Check sheet for the modelled part. Datum: model origin and axes. Units: mm. Round coordinates to 2 decimals unless told otherwise and drop trailing zeros. Write each loop counter-clockwise with the first axis right and the second up, starting at its lowest first coordinate (ties: lowest second). Pieces come first, ordered by that corner, then holes. Notation, with made-up numbers: (-21.5, 89) -> (-10.5, 89) arc R6 cw to (-10.5, 98) -> close; hole circle Ø11 at (63, 26.25). An arc over 180 degrees is marked (long way). One line per item, written item: value.
Autodesk Inventor part; units mm, degrees
ref_plane "YZ Plane" through (0, 0, 0) normal (1, 0, 0) x (0, 1, 0)
ref_plane "XZ Plane" through (0, 0, 0) normal (0, 1, 0) x (-1, 0, 0)
ref_plane "XY Plane" through (0, 0, 0) normal (0, 0, 1) x (1, 0, 0)
sketch "Sketch1" plane through (0, 0, 0) normal (0, 1, 0) x (-1, 0, 0)
  line L0 (45, -45) -> (-45, -45)
  line L1 (-45, -45) -> (-45, 45)
  line L2 (-45, 45) -> (45, 45)
  line L3 (45, 45) -> (45, -45)
  line L4 (45, -45) -> (-45, 45) construction
  line L5 (-45, -45) -> (45, 45) construction
  point P0 (0, 0)
  dimension "d2" = 90
  dimension "d3" = 90
extrude "Extrusion1" add sketch "Sketch1" along normal blind 2
sketch "Sketch2" plane through (0, 2, 0) normal (0, 1, 0) x (1, 0, 0)
  line L0 (45, -45) -> (45, 45)
  line L1 (45, 45) -> (41, 45)
  line L2 (45, 45) -> (-45, 45)
  circle A0 centre (41, 41) radius 2
  point P0 (0, 0)
hole "Hole1" at (41, 2, -41) direction (0, -1, 0) diameter 4 end through all
sketch "Sketch3" plane through (0, 2, 0) normal (0, 1, 0) x (1, 0, 0)
  circle A0 centre (-41, 41) radius 2
  line L0 (-45, 45) -> (-45, -45)
  circle A1 centre (-41, -41) radius 2
  line L1 (45, -45) -> (45, 45)
  circle A2 centre (41, -41) radius 2
  point P0 (0, 0)
  dimension "d17" = 4
  dimension "d21" = 4
extrude "Extrusion2" cut sketch "Sketch3" against normal blind 2
fillet "Fillet1" radius 3.5 4 edges at (-45, 1, -45) (45, 1, -45) (45, 1, 45) (-45, 1, 45)
sketch "Sketch5" plane through (0, 2, 0) normal (0, 1, 0) x (1, 0, 0)
  line L0 (40, 40) -> (-40, 40)
  line L1 (-40, 40) -> (-40, -40)
  line L2 (-40, -40) -> (40, -40)
  line L3 (40, -40) -> (40, 40)
  line L4 (40, 40) -> (-40, -40) construction
  line L5 (-40, 40) -> (40, -40) construction
  line L6 (-9.8412, 41.25) -> (-37.3412, 41.25)
  line L7 (-37.3412, 41.25) -> (-37.3412, -41.25)
  line L8 (-37.3412, -41.25) -> (-9.8412, -41.25)
  line L9 (-9.8412, -41.25) -> (-9.8412, 41.25)
  line L10 (-9.8412, 41.25) -> (-37.3412, -41.25) construction
  line L11 (-37.3412, 41.25) -> (-9.8412, -41.25) construction
  line L12 (26.1588, 41.25) -> (-6.3412, 41.25)
  line L13 (-6.3412, 41.25) -> (-6.3412, -41.25)
  line L14 (-6.3412, -41.25) -> (26.1588, -41.25)
  line L15 (26.1588, -41.25) -> (26.1588, 41.25)
  line L16 (26.1588, 41.25) -> (-6.3412, -41.25) construction
  line L17 (-6.3412, 41.25) -> (26.1588, -41.25) construction
  line L18 (37.1268, 41.25) -> (29.6588, 41.25)
  line L19 (29.6588, 41.25) -> (29.6588, -41.25)
  line L20 (29.6588, -41.25) -> (37.1268, -41.25)
  line L21 (37.1268, -41.25) -> (37.1268, 41.25)
  line L22 (37.1268, 41.25) -> (29.6588, -41.25) construction
  line L23 (29.6588, 41.25) -> (37.1268, -41.25) construction
  line L24 (-41.5049, 41.25) -> (-37.5049, 41.25)
  line L25 (41.2164, 37.1336) -> (36.7164, 37.1336)
  line L26 (36.7164, 37.1336) -> (36.7164, -36.7164)
  line L27 (36.7164, -36.7164) -> (41.2164, -36.7164)
  line L28 (41.2164, -36.7164) -> (41.2164, 37.1336)
  line L29 (41.2164, 37.1336) -> (36.7164, -36.7164) construction
  line L30 (36.7164, 37.1336) -> (41.2164, -36.7164) construction
  line L31 (37.1268, 41.25) -> (41.1268, 41.25)
  line L32 (41.1268, 41.25) -> (41.1268, 37.25)
  point P0 (0, 0)
  point P1 (-23.5912, 0)
  point P2 (9.9088, 0)
  point P3 (33.3928, 0)
  point P4 (38.9664, 0.2086)
  point P5 (37.1268, 37.1336)
  point P6 (37.1268, 40)
  point P7 (29.6588, 40)
  point P8 (29.6588, -40)
  point P9 (37.1268, -40)
  point P10 (37.1268, -36.7164)
  dimension "d25" = 80
  dimension "d26" = 80
  dimension "d27" = 27.5
  dimension "d28" = 82.5
  dimension "d29" = 32.5
  dimension "d30" = 82.5
  dimension "d31" = 7.468
  dimension "d32" = 82.5
  dimension "d33" = 4
  dimension "d34" = 3.5
  dimension "d35" = 3.5
  dimension "d36" = 4.5
  dimension "d37" = 4
  dimension "d38" = 4
  dimension "d39" = 73.85
extrude "Extrusion4" cut sketch "Sketch5" against normal through all contours L21 L25 L26 L27 L2 L19 L0 | L0 L19 L18 L21 | L25 L28 L27 L3 | L3 L27 L21 L25 | L21 L27 L26 L25 | L15 L2 L13 L0 | L0 L13 L12 L15 | L2 L21 L20 L19 | L15 L14 L13 L2 | L9 L2 L7 L0 | L0 L7 L6 L9 | L9 L8 L7 L2
sketch "Sketch8" plane through (0, 2, 0) normal (0, 1, 0) x (1, 0, 0)
  line L0 (-45, 41.5) -> (-45, -41.5)
  line L1 (-45, 41.5) -> (-44, 41.5)
  line L2 (41.5, 45) -> (-41.5, 45)
  line L3 (-41.5, 45) -> (-41.5, 44)
  line L4 (-45, -41.5) -> (-44, -41.5)
  arc A0 (-45, -41.5) -> (-41.5, -45) centre (-41.5, -41.5) ccw
  line L5 (-41.5, -45) -> (-41.5, -44)
  line L6 (41.5, -45) -> (41.5, -44)
  arc A1 (41.5, -45) -> (45, -41.5) centre (41.5, -41.5) ccw
  line L7 (45, -41.5) -> (44, -41.5)
  arc A2 (45, 41.5) -> (41.5, 45) centre (41.5, 41.5) ccw
  circle A3 centre (-41, -41) radius 2
  line L8 (-41, -39) -> (-41, -38)
  line L9 (-39, -41) -> (-38, -41)
  circle A4 centre (-41, 41) radius 2
  line L10 (-39, 41) -> (-38, 41)
  line L11 (-41, 39) -> (-41, 38)
  circle A5 centre (41, 41) radius 2
  line L12 (37.1268, 41.25) -> (37.1268, 37.1336)
  circle A6 centre (41, -41) radius 2
  line L13 (41, -39) -> (41, -38)
  line L14 (39, -41) -> (38, -41)
  line L15 (-44, 37.3438) -> (-41.5, 37.3438)
  line L16 (-41.5, 37.3438) -> (-41.5, -37.5309)
  line L17 (-41.5, -37.5309) -> (-44, -37.5309)
  line L18 (-44, -37.5309) -> (-44, 37.3438)
  line L19 (37.5845, -44) -> (-37.7671, -44)
  line L20 (-37.7671, -44) -> (-37.7671, -41.5)
  line L21 (-37.7671, -41.5) -> (37.5845, -41.5)
  line L22 (37.5845, -41.5) -> (37.5845, -44)
  line L23 (44, 34.9904) -> (41.5, 34.9904)
  line L24 (41.5, 34.9904) -> (41.5, -37.4955)
  line L25 (41.5, -37.4955) -> (44, -37.4955)
  line L26 (44, -37.4955) -> (44, 34.9904)
  line L27 (-37.4232, 44) -> (37.7379, 44)
  line L28 (37.7379, 44) -> (37.7379, 41.5)
  line L29 (37.7379, 41.5) -> (-37.4232, 41.5)
  line L30 (-37.4232, 41.5) -> (-37.4232, 44)
  line L31 (26.1588, -41.5) -> (28.1588, -41.5)
  line L32 (28.1588, -41.5) -> (28.1588, 41.5)
  line L33 (28.1588, 41.5) -> (26.1588, 41.5)
  line L34 (26.1588, 41.5) -> (26.1588, -41.5)
  line L35 (-9.8412, -41.5) -> (-7.8412, -41.5)
  line L36 (-7.8412, -41.5) -> (-7.8412, 41.5)
  line L37 (-7.8412, 41.5) -> (-9.8412, 41.5)
  line L38 (-9.8412, 41.5) -> (-9.8412, -41.5)
  point P0 (0, 0)
  dimension "d46" = 1
  dimension "d47" = 1
  dimension "d48" = 1
  dimension "d49" = 1
  dimension "d50" = 1
  dimension "d51" = 1
  dimension "d54" = 1
  dimension "d55" = 1
  dimension "d56" = 1
  dimension "d57" = 1
  dimension "d60" = 1
  dimension "d61" = 1
  dimension "d63" = 2.5
  dimension "d64" = 2.5
  dimension "d65" = 2.5
  dimension "d72" = 2
  dimension "d73" = 2
extrude "Extrusion5" add sketch "Sketch8" along normal blind 5 contours L15 L16 L17 L18 | L19 L20 L21 L22 | L21 L34 L29 L32 | L38 L29 L36 L21 | L29 L30 L27 L28 | L26 L25 L24 L23
fillet "Fillet3" radius 3.5 1 edges at (37.1268, 1, 36.7164)
fillet "Fillet4" radius 3.5 8 edges at (-6.3412, 1, 41.25) (-6.3412, 1, -41.25) (29.6588, 1, -41.25) (29.6588, 1, 41.25) (26.1588, 1, -41.25) (-9.8412, 1, -41.25) (26.1588, 1, 41.25) (-9.8412, 1, 41.25)
fillet "Fillet7" radius 1 4 edges at (-7.8412, 4.5, 41.5) (28.1588, 4.5, 41.5) (26.1588, 4.5, 41.5) (-9.8412, 4.5, 41.5)
sketch "Sketch10" plane through (0, 0, 0) normal (0, -1, 0) x (1, 0, 0)
  line L0 (-37.3412, -41.25) -> (-37.3412, 41.25)
  line L1 (-37.3412, 37.75) -> (-40.8412, 37.75)
  line L2 (-40.8412, 37.75) -> (-40.8412, -37)
  line L3 (-40.8412, -37) -> (-37.3412, -37)
  line L4 (-37.3412, -37) -> (-37.3412, 37.75)
  point P0 (0, 0)
  point P1 (-37.3412, -37.75)
  dimension "d78" = 3.5
extrude "Extrusion6" cut sketch "Sketch10" against normal through all
fillet "Fillet8" radius 3.5 1 edges at (-37.3412, 1, -37)
fillet "Fillet11" radius 3.5 2 edges at (37.1268, 1, -37.1336) (-37.3412, 1, 37.75)
sketch "Sketch19" plane through (-37.7671, 2, 44) normal (0, 0, 1) x (1, 0, 0)
  line L0 (75.3516, 0) -> (0, 0)
  line L1 (0, 5) -> (75.3516, 5)
  line L2 (0, 0) -> (0, 5)
  line L3 (0, 5) -> (0, 3)
  line L4 (0, 3) -> (1.2108, 3)
  line L5 (1.2108, 3) -> (1.2108, 5)
  line L6 (1.2108, 5) -> (0, 5)
  line L7 (0, 5) -> (0, 3)
  point P0 (37.7671, -2)
  dimension "d90" = 2
  dimension "d106" = 1.2108
extrude "Extrusion7" cut sketch "Sketch19" against normal blind 3
sketch "Sketch21" plane through (25.1588, 2, 41.5) normal (0, 0, -1) x (-1, 0, 0)
  line L0 (32, 0) -> (0, 0)
  line L1 (0, 5) -> (32, 5)
  line L2 (28.159, 5) -> (29.959, 5)
  line L3 (29.959, 5) -> (29.959, 4)
  line L4 (28.159, 5) -> (26.359, 5)
  line L5 (29.959, 5) -> (26.359, 5)
  line L6 (26.359, 5) -> (26.359, 3)
  line L7 (26.359, 3) -> (29.959, 3)
  line L8 (29.959, 3) -> (29.959, 5)
  point P0 (25.1588, -2)
  point P1 (29.959, 4)
  dimension "d102" = 1.8
  dimension "d103" = 1
  dimension "d104" = 1.8
  dimension "d105" = 2
extrude "Extrusion8" cut sketch "Sketch21" against normal up to surface (2.5 mm away)
sketch "Sketch22" plane through (-9.8412, 2, -41.5) normal (-1, 0, 0) x (0, 0, 1)
  line L0 (0, 5) -> (82, 5)
  line L1 (0, 5) -> (3, 5)
  line L2 (3.75, 0) -> (0, 0)
  line L3 (3, 5) -> (0, 5)
  line L4 (0, 5) -> (0, 0)
  line L5 (0, 0) -> (3, 0)
  line L6 (3, 0) -> (3, 5)
  point P0 (41.5, -2)
  point P1 (3, 0)
  dimension "d98" = 3
extrude "Extrusion9" cut sketch "Sketch22" against normal up to surface (38 mm away)
sketch "Sketch23" plane through (-37.7671, 2, 44) normal (0, 0, 1) x (1, 0, 0)
  line L0 (33.7518, 5) -> (31.9518, 5)
  line L1 (36.5669, 5) -> (75.3516, 5)
  line L2 (31.9518, 5) -> (31.9518, 3.1171)
  point P0 (37.7671, -2)
  point P1 (0.3379, 5)
  dimension "d101" = 1.8
sketch "Sketch24" plane through (-37.7671, 2, 44) normal (0, 0, 1) x (1, 0, 0)
  point P0 (37.7671, -2)
properties part number "LeftCover" material "ABS Plastic"
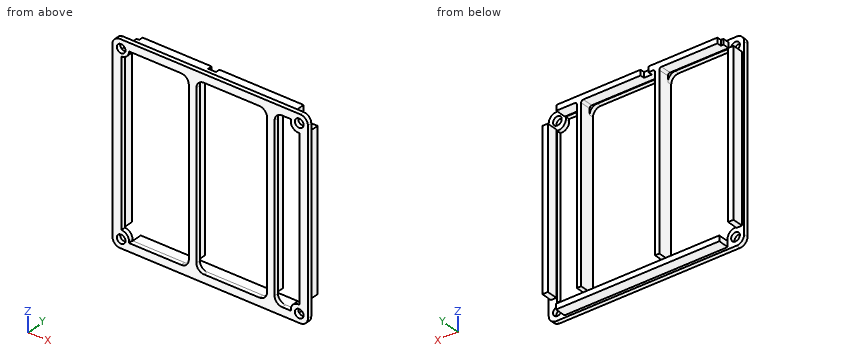
Item 1: Sectioned sample at B-B on x = 18. Enter the section's corners in (y, z), and give its area (3 significant figures).
Answer:
outline: (0, -45) -> (2, -45) -> (2, -44) -> (7, -44) -> (7, -41.5) -> (2, -41.5) -> (2, -41.25) -> (0, -41.25) -> close; (0, 41.25) -> (2, 41.25) -> (2, 41.5) -> (7, 41.5) -> (7, 44) -> (2, 44) -> (2, 45) -> (0, 45) -> close
area: 40.0 mm^2
Item 2: Depth check by flat-ended pin: P1, Ø6, axis at x = -35.5, z = -0.5, coming from the +Y side (3 decimals); P2, Ø1.2, axis at y = 3.5, z = -42.5, coming from the -X side; P3, Ø2, axis at x = -42.5, y = 3.5, coming from the -Z side; P4, Ø0.6, axis at x = -8.5, y = 4, coming from the -Z side. Enter the tip coordinate at first touch or a pass-through.
Answer:
P1: passes through
P2: stops at x = -37.42
P3: stops at z = -37.34
P4: stops at z = -44
Item 3: Thickness scan on line 1 (X direction, y = 5, z = 25); line 2 (Z direction, x = -41, y = 1); line 3 (Z direction, x = 41, y = 1.55). Record the ranges inside material, lowest first.
Answer:
line 1: x = -44 to -41.5, -9.84 to -7.84, 26.16 to 28.16, 41.5 to 44
line 2: z = -45 to -43, -39 to 39, 43 to 45
line 3: z = -45 to -43, -39 to -37.13, 36.72 to 39, 43 to 45
Item 4: Sectioned sample at A-A on z = 24. Enter the section's corners in (x, y), and give its area (3 significant figures).
Answer:
outline: (-45, 0) -> (-40.84, 0) -> (-40.84, 2) -> (-41.5, 2) -> (-41.5, 7) -> (-44, 7) -> (-44, 2) -> (-45, 2) -> close; (-9.84, 0) -> (-6.34, 0) -> (-6.34, 2) -> (-7.84, 2) -> (-7.84, 7) -> (-9.84, 7) -> close; (26.16, 0) -> (29.66, 0) -> (29.66, 2) -> (28.16, 2) -> (28.16, 7) -> (26.16, 7) -> close; (41.22, 0) -> (45, 0) -> (45, 2) -> (44, 2) -> (44, 7) -> (41.5, 7) -> (41.5, 2) -> (41.22, 2) -> close
area: 74.9 mm^2
